Work out the finished part from the listing and answer in its coordinate system (mm). A direction names the side the tool comes from. Coordinates: 2 decimals unless noted, no trailing zeros. Write each loop counter-clockwise with the first axis right and the second up, starting at its lowest first coordinate (ties: lowest second). Pieces come first, ordered by that corner, then holes. Notation, with made-up numbers: (69, 79.25) - (99, 79.25) arc R6 cw to (99, 90.25) - close; hole circle Ø11 at (-29.5, -21). An arc over 180 degrees is marked (long way). Use one line per item in the form item = value. Start each with the question number.
Item 1: Given pin 1 (8 mm diameter, centred on y = 18, z = -16.5, fed in from +X); pin 2 (3 mm diameter, centred on x = -20.5, y = 19, fed in from -Z); pin 3 (1.2 mm diameter, centred on y = 19.5, z = -4, fed in from +X), each flat-ended and moving along its own axis, determine where each tip first touches the part or whether it passes through.
Item 2: A cutting plane is placed at A-A (z = -3.5). Give the number of separate pieces and of enclosed holes in the cut face, then the cut area to 3 significant figures.
Item 3: For faces 5 (the flat face through (22.796, 19, -3)), 6 (the cylindrical face through (27.292, 2.465, -2.812)), 7 (the flat face through (-22, 19, -10.114)), 8 (the flat face through (16.6, 17.5, -4.4)), determine the directions among +Z, -Z, +X, -X, +Y, -Y from which every point of the face is accessible in a straight line to the end or side of a thin tool.
Item 4: Consider probe 1 along X at (y, z) = (2.75, 1.5); probe 2 along Y at (x, z) = (-29, 14); probe 3 along X at (y, z) = (7.25, 6). Determine where each line is inside the solid, lowest interval first.
Item 5: A cutting plane is placed at D-D (z = 3). Write down the section's boundary in (x, y).
Item 6: Determine the mould class of faces 1 (the flat face through (18, 19, 4.886)), 2 (the cylindrical face through (-2.429, 9.752, -2.334)), 3 (the flat face through (32.796, 2, -2)), 4 (the flat face through (-37.204, 2, -2)) for opening direction X: released by +X, released by -X, zero draft, split by the parting line, or undercut.
Item 7: A cutting plane is placed at B-B (y = 10.75). Write down the section's boundary in (x, z).
Item 8: A cutting plane is placed at C-C (x = 21.5). Write down the section's boundary in (y, z).
from build123d import *

# Parameters (mm, degrees)
SKETCH1_W                = 70
SKETCH1_H                = 40
BOSS_EXTRUDE1_DEPTH      = 5
SKETCH2_W                = 30
SKETCH2_H                = 40
BOSS_EXTRUDE2_DEPTH      = 15
SKETCH3_R                = 10.25
CUT_EXTRUDE1_DEPTH       = 41
SKETCH5_W                = 10
SKETCH5_H                = 15
BOSS_EXTRUDE3_DEPTH      = 2.5
SKETCH6_W                = 10
SKETCH6_H                = 15
BOSS_EXTRUDE4_DEPTH      = 2.5
M3_CLEARANCE_HOLE1_D     = 3.4
M3_CLEARANCE_HOLE1_DEPTH = 2.5
M8_CLEARANCE_HOLE1_D     = 9
M8_CLEARANCE_HOLE1_DEPTH = 5


with BuildPart() as part:
    # Sketch1 → Boss-Extrude1 (new body)
    with BuildSketch(Plane(origin=(0, 0, 0), x_dir=(1, 0, 0), z_dir=(0, 1, 0))):
        with Locations((-2.203647416, 2.613981763)):
            Rectangle(SKETCH1_W, SKETCH1_H)
    extrude(amount=BOSS_EXTRUDE1_DEPTH)

    # Sketch2 → Boss-Extrude2 (add)
    with BuildSketch(Plane(origin=(0, 5, 0), x_dir=(1, 0, 0), z_dir=(0, 1, 0))):
        with Locations((-2.203647416, 2.613981763)):
            Rectangle(SKETCH2_W, SKETCH2_H)
    extrude(amount=BOSS_EXTRUDE2_DEPTH)

    # Sketch3 → Cut-Extrude1 (cut, through all)
    with BuildSketch(Plane.XY.offset(17.386018237)):
        with Locations((-2.203647416, 20)):
            Circle(SKETCH3_R)
    extrude(amount=-CUT_EXTRUDE1_DEPTH, mode=Mode.SUBTRACT)

    # Sketch5 → Boss-Extrude3 (add)
    with BuildSketch(Plane(origin=(0, 20, 0), x_dir=(1, 0, 0), z_dir=(0, 1, 0))):
        with Locations((-22.203647416, 2.613981763)):
            Rectangle(SKETCH5_W, SKETCH5_H)
    extrude(amount=-BOSS_EXTRUDE3_DEPTH)

    # Sketch6 → Boss-Extrude4 (add)
    with BuildSketch(Plane(origin=(0, 20, 0), x_dir=(1, 0, 0), z_dir=(0, 1, 0))):
        with Locations((17.796352584, 2.613981763)):
            Rectangle(SKETCH6_W, SKETCH6_H)
    extrude(amount=-BOSS_EXTRUDE4_DEPTH)

    # M3 Clearance Hole1
    with Locations(Plane(origin=(0, 20, 0), x_dir=(1, 0, 0), z_dir=(0, 1, 0))):
        with Locations((17.796352584, 2.613981763), (-22.203647416, 2.613981763)):
            Hole(M3_CLEARANCE_HOLE1_D / 2, depth=M3_CLEARANCE_HOLE1_DEPTH)

    # M8 Clearance Hole1
    with Locations(Plane(origin=(0, 5, 0), x_dir=(1, 0, 0), z_dir=(0, 1, 0))):
        with Locations((22.796352584, 2.613981763), (-27.203647416, 2.613981763)):
            Hole(M8_CLEARANCE_HOLE1_D / 2, depth=M8_CLEARANCE_HOLE1_DEPTH)


solid = part.part
Answer:
q1.pin_1 = 12.8
q1.pin_2 = -10.11
q1.pin_3 = 22.8
q2.separate_pieces = 5
q2.enclosed_holes = 0
q2.area = 582 mm²
q3.face_5 = +Z, -Z, +X, +Y
q3.face_6 = -Y
q3.face_7 = -Z, -X, +Y
q3.face_8 = +Z, -Z, +X
q4.probe_1 = -37.2 to -29.03, -25.38 to 20.97, 24.62 to 32.8
q4.probe_2 = 0 to 5
q4.probe_3 = -17.2 to 12.8
q5.outline = (-37.2, 0) - (32.8, 0) - (32.8, 5) - (12.8, 5) - (12.8, 17.5) - (22.8, 17.5) - (22.8, 20) - (8.05, 20) arc R10.25 cw to (-12.45, 20) - (-27.2, 20) - (-27.2, 17.5) - (-17.2, 17.5) - (-17.2, 5) - (-37.2, 5) - close
q6.face_1 = zero draft
q6.face_2 = undercut
q6.face_3 = released by +X
q6.face_4 = released by -X
q7.outline = (-17.2, -22.61) - (-6.62, -22.61) - (-6.62, 17.39) - (-17.2, 17.39) - close; (2.21, -22.61) - (12.8, -22.61) - (12.8, 17.39) - (2.21, 17.39) - close
q8.outline = (0, -22.61) - (5, -22.61) - (5, -6.92) - (0, -6.92) - close; (0, 1.7) - (5, 1.7) - (5, 17.39) - (0, 17.39) - close; (17.5, -10.11) - (20, -10.11) - (20, 4.89) - (17.5, 4.89) - close
